The listing builds one solid part. Answer for the finished solid, in the listing's coordinates (mm). A direction names the side the tool comes from. Give positions to 0.01 mm unless a question says otherwise; leave off trailing zeros. Write each loop counter-clockwise with the first axis right and the second up, starting at its lowest first coordinate (ties: lowest second). Pieces come first, ordered by that corner, then holes. Notation, with made-up numbers: (-35, -19) - (-6, -19) arc R16 cw to (-6, -1) - close; hole circle Ø8 at (82.25, 3.25). An arc over 180 degrees is marked (long way). Write each question's results on one line, items separated by ' | '. Start each with the question number.
Q1. For faces 4 (the face through (-15.891, -12.526, 8.987)), 5 (the face through (-13.97, 33.59, 9.37)), 6 (the face through (14.03, 28.41, 9.37)), 7 (the face through (-10, 31, 19)), determine the directions among +Z, -Z, +X, -X, +Y, -Y from which every point of the face is accessible in a straight line to the end or side of a thin tool.
Q2. Section C-C (z = 24.5) is taken. Determine the outline of the cut face in (x, y), plus the area to 3 significant figures.
Q3. For a pull along X with two mould halves and no side action, classify faces 1 (the face through (15.109, -12.526, 8.987)), 2 (the face through (0, 20, 36.5)), 3 (the face through (12, 33, 4)) as pulls with the +X half, pulls with the -X half, needs draft (parallel to the pull), parting line crosses it, or undercut.
Q4. Section B-B (y = 7.5) is taken. Determine the outline of the cut face in (x, z), plus the area to 3 significant figures.
Q5. Flat-ended cylindrical pins translate along their axes: pin 1 Ø5 at (x, y) = (-15.5, 15.5) entering from +Z; pin 2 Ø7.5 at (y, z) = (31, 6) entering from -X; pin 3 Ø12 at (x, z) = (1, 17) entering from +Y; pin 4 Ø8 at (x, y) = (-11.5, -2.5) entering from -Z. Find the tip coordinate at first contact, or state that the pin passes through.
Q6. Section D-D (x = -8.5) is taken. Determine the outline of the cut face in (y, z), plus the area to 3 significant figures.
Q7. Find the intervals of material crossed by probe 1 along Z at (x, y) = (11.25, 31); probe 2 along X at (y, z) = (15.5, 1.95); probe 3 along Y at (x, z) = (15.5, 1.7), in increasing order.
Q8. Section A-A (x = 1.5) is taken. Determine the outline of the cut face in (y, z), plus the area to 3 significant figures.
```python
from build123d import *

# Parameters (mm, degrees)
SKETCH_1_W               = 42
SKETCH_1_H               = 42
EXTRUDE_1_DEPTH          = 6.5
EXTRUDE_2_DEPTH          = 42
SKETCH_2_R               = 15
CUT_EXTRUDE_2_DEPTH      = 57.870466852
SKETCH_4_R               = 1.75
CUT_EXTRUDE_1_DEPTH      = 57.870466852
CHAMFER_1_SIZE           = 5
CUT_EXTRUDE_3_DEPTH      = 68.507407001
SKETCH_7_R               = 3
CUT_EXTRUDE_4_DEPTH      = 31.5
CUT_EXTRUDE_5_DEPTH      = 48.055817919
CUT_EXTRUDE_5_DEPTH_BACK = 5
SKETCH_8_R               = 2.6
SKETCH_9_R               = 4.25
CUT_EXTRUDE_6_DEPTH      = 18.5
SKETCH_10_R              = 15
SKETCH_10_R_2            = 11.5
EXTRUDE_3_DEPTH          = 3
SKETCH_11_W              = 6
SKETCH_11_H              = 36.5
EXTRUDE_4_DEPTH          = 20
CUT_EXTRUDE_7_DEPTH      = 67.198564994
CUT_EXTRUDE_7_DEPTH_BACK = 67.198564994
SKETCH_12_R              = 2.6
SKETCH_13_R              = 4.25
CUT_EXTRUDE_8_DEPTH      = 4
CUT_EXTRUDE_START        = -4
SKETCH_14_R              = 4.25
CUT_EXTRUDE_9_DEPTH      = 4


with BuildPart() as part:
    # 草圖1 → 填料-伸長1 (new body)
    with BuildSketch(Plane.XY):
        Rectangle(SKETCH_1_W, SKETCH_1_H)
    extrude(amount=EXTRUDE_1_DEPTH)

    # 草圖5 → 填料-伸長2 (add)
    with BuildSketch(Plane(origin=(21, 0, 0), x_dir=(0, 0, -1), z_dir=(1, 0, 0))):
        Polygon((-6.5, -21), (-48.5, 21), (-6.5, 21), align=None)
    extrude(amount=-EXTRUDE_2_DEPTH)

    # 草圖2 → 除料-伸長2 (cut, through all)
    with BuildSketch(Plane.XY):
        with Locations(Location((0, 0, 0), (0, 0, 270))):
            Circle(SKETCH_2_R)
    extrude(amount=CUT_EXTRUDE_2_DEPTH, mode=Mode.SUBTRACT)

    # 草圖4 → 除料-伸長1 (cut, through all)
    with BuildSketch(Plane.XY):
        with Locations(Location((-15.5, 15.5, 0), (0, 0, 270))):
            Circle(SKETCH_4_R)
        with Locations(Location((-15.5, -15.5, 0), (0, 0, 180))):
            Circle(SKETCH_4_R)
        with Locations(Location((15.5, -15.5, 0), (0, 0, 270))):
            Circle(SKETCH_4_R)
        with Locations(Location((15.5, 15.5, 0), (0, 0, 180))):
            Circle(SKETCH_4_R)
    extrude(amount=CUT_EXTRUDE_1_DEPTH, mode=Mode.SUBTRACT)

    # 導角1
    chamfer_1_edges = [part.edges().sort_by_distance(p)[0] for p in [
        (-21, 21, 24.25),
        (21, 21, 24.25),
        (21, -21, 3.25),
        (-21, -21, 3.25),
    ]]
    chamfer(chamfer_1_edges, length=CHAMFER_1_SIZE)

    # 草圖6 → 除料-伸長3 (cut, through all)
    with BuildSketch(Plane.ZY.offset(21)):
        Polygon((48.5, 21), (36.5, 21), (36.5, 9), align=None)
    extrude(amount=-CUT_EXTRUDE_3_DEPTH, mode=Mode.SUBTRACT)

    # 草圖7 → 除料-伸長4 (cut)
    with BuildSketch(Plane.XY.offset(36.5)):
        with Locations((-15.5, 15.5)):
            Circle(SKETCH_7_R)
        with Locations((15.5, 15.5)):
            Circle(SKETCH_7_R)
        with Locations((15.5, -15.5)):
            Circle(SKETCH_7_R)
        with Locations((-15.5, -15.5)):
            Circle(SKETCH_7_R)
    extrude(amount=-CUT_EXTRUDE_4_DEPTH, mode=Mode.SUBTRACT)

    # 草圖8 → 除料-伸長5 (cut, two sides: drawn at the far end of the back side and taken through both)
    with BuildSketch(Plane(origin=(0, 0, 0), x_dir=(1, 0, 0), z_dir=(0, 1, 0)).offset(-CUT_EXTRUDE_5_DEPTH_BACK)):
        with Locations(Location((0, -15, 0), (0, 0, 90))):
            Circle(SKETCH_8_R)
        with Locations(Location((0, -31, 0), (0, 0, 90))):
            Circle(SKETCH_8_R)
    extrude(amount=CUT_EXTRUDE_5_DEPTH + CUT_EXTRUDE_5_DEPTH_BACK, mode=Mode.SUBTRACT)

    # 草圖9 → 除料-伸長6 (cut)
    with BuildSketch(Plane(origin=(0, 0, 0), x_dir=(1, 0, 0), z_dir=(0, 1, 0))):
        with Locations(Location((0, -31, 0), (0, 0, 90))):
            Circle(SKETCH_9_R)
        with Locations(Location((0, -15, 0), (0, 0, 90))):
            Circle(SKETCH_9_R)
    extrude(amount=CUT_EXTRUDE_6_DEPTH, mode=Mode.SUBTRACT)

    # 草圖10 → 填料-伸長3 (add)
    with BuildSketch(Plane(origin=(0, 0, 0), x_dir=(-1, 0, 0), z_dir=(0, 0, -1))):
        Circle(SKETCH_10_R)
        Circle(SKETCH_10_R_2, mode=Mode.SUBTRACT)
    extrude(amount=-EXTRUDE_3_DEPTH)

    # 草圖11 → 填料-伸長4 (add)
    with BuildSketch(Plane(origin=(0, 21, 0), x_dir=(1, 0, 0), z_dir=(0, 1, 0))):
        with Locations((13, -18.25)):
            Rectangle(SKETCH_11_W, SKETCH_11_H)
        with Locations((-13, -18.25)):
            Rectangle(SKETCH_11_W, SKETCH_11_H)
    extrude(amount=EXTRUDE_4_DEPTH)

    # 草圖12 → 除料-伸長7 (cut, two sides: drawn at the far end of the back side and taken through both)
    with BuildSketch(Plane(origin=(16, 0, 0), x_dir=(0, 0, -1), z_dir=(1, 0, 0)).offset(-CUT_EXTRUDE_7_DEPTH_BACK)):
        with Locations((-30.5, 31)):
            Circle(SKETCH_12_R)
        with Locations((-6, 31)):
            Circle(SKETCH_12_R)
    extrude(amount=CUT_EXTRUDE_7_DEPTH + CUT_EXTRUDE_7_DEPTH_BACK, mode=Mode.SUBTRACT)

    # 草圖13 → 除料-伸長8 (cut)
    with BuildSketch(Plane(origin=(16, 0, 0), x_dir=(0, 0, -1), z_dir=(1, 0, 0))):
        with Locations((-30.5, 31)):
            Circle(SKETCH_13_R)
        with Locations((-6, 31)):
            Circle(SKETCH_13_R)
    extrude(amount=-CUT_EXTRUDE_8_DEPTH, mode=Mode.SUBTRACT)

    # 草圖14 → 除料-伸長9 (cut)
    with BuildSketch(Plane.ZY.offset(16).offset(CUT_EXTRUDE_START)):
        with Locations(Location((30.5, 31, 0), (0, 0, 180))):
            Circle(SKETCH_14_R)
        with Locations(Location((6, 31, 0), (0, 0, 180))):
            Circle(SKETCH_14_R)
    extrude(amount=CUT_EXTRUDE_9_DEPTH, mode=Mode.SUBTRACT)


solid = part.part
```
Answers below:
1) face 4: +Z | face 5: -X | face 6: +X | face 7: +Z, -Z, +Y
2) outline: (-21, -3) - (-14.7, -3) arc R15 cw (long way) to (14.7, -3) - (21, -3) - (21, 16) - (16, 21) - (16, 41) - (10, 41) - (10, 21) - (-10, 21) - (-10, 41) - (-16, 41) - (-16, 21) - (-21, 16) - close; hole circle Ø6 at (-15.5, 15.5); hole circle Ø6 at (15.5, 15.5) | area: 724 mm2
3) face 1: undercut | face 2: needs draft | face 3: pulls with the +X half
4) outline: (-21, 0) - (-8.72, 0) - (-8.72, 3) - (-12.99, 3) - (-12.99, 35) - (-21, 35) - close; (8.72, 0) - (21, 0) - (21, 35) - (12.99, 35) - (12.99, 3) - (8.72, 3) - close | area: 586 mm2
5) pin 1: stops at z = 5 | pin 2: stops at x = -12 | pin 3: stops at y = 21 | pin 4: stops at z = 0
6) outline: (-21, 0) - (-7.75, 0) - (-7.75, 3) - (-12.36, 3) - (-12.36, 15.14) - (-21, 6.5) - close; (7.75, 0) - (21, 0) - (21, 36.5) - (12.36, 36.5) - (12.36, 3) - (7.75, 3) - close | area: 437 mm2
7) probe 1: z = 0 to 3.4, 8.6 to 27.9, 33.1 to 36.5 | probe 2: x = -21 to -17.25, -13.75 to 13.75, 17.25 to 21 | probe 3: y = -21 to -17.25, -13.75 to 13.75, 17.25 to 41
8) outline: (-21, 0) - (-11.4, 0) - (-11.4, 3) - (-14.92, 3) - (-14.92, 12.58) - (-21, 6.5) - close; (11.4, 0) - (21, 0) - (21, 12.88) - (18.5, 12.88) - (18.5, 11.02) - (14.92, 11.02) - (14.92, 3) - (11.4, 3) - close; (14.92, 18.98) - (18.5, 18.98) - (18.5, 17.12) - (21, 17.12) - (21, 28.88) - (18.5, 28.88) - (18.5, 27.02) - (14.92, 27.02) - close; (14.92, 34.98) - (18.5, 34.98) - (18.5, 33.12) - (21, 33.12) - (21, 36.5) - (14.92, 36.5) - close | area: 223 mm2
